Geometry: see drawing. Coordinates: mm, zero at the bounding-box minimum. Coordinates: 2 decimals unless noted, no trailing zeros. Loops run counter-clockwise (first coordinate to the right, second up) from the corner with the lowest first, then second, coordinate; pieces in that order, holes last.
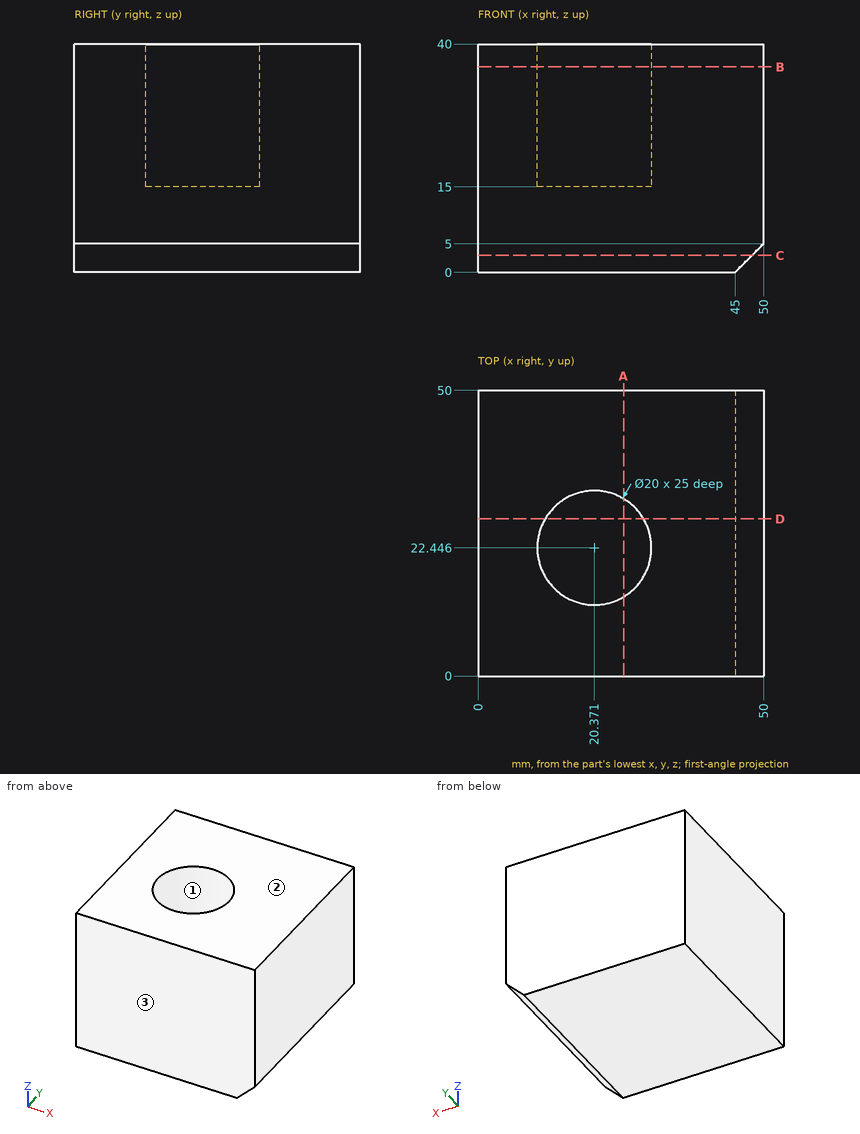
Item 1: Section query B-B (z = 36). Output: boundary loops of the cut face in (x, y) (1 decimal), then the cut area to 3 significant figures.
Result:
outline: (0, 0) - (50, 0) - (50, 50) - (0, 50) - close; hole circle Ø20 at (20.4, 22.4)
area: 2,190 mm2
Item 2: Section query D-D (y = 27.5). Output: boundary loops of the cut face in (x, z), then the cut area to 3 significant figures.
Result:
outline: (0, 0) - (45, 0) - (50, 5) - (50, 40) - (29, 40) - (29, 15) - (11.74, 15) - (11.74, 40) - (0, 40) - close
area: 1,560 mm2
Item 3: Mould query, pull axis Y, two halves, no side actions, for the marked faces 1, 2 and 3. Classes: +Y half, -Y half, draft (parallel to the pull), parting line (faces both ways), or undercut.
Result:
face 1: undercut
face 2: draft
face 3: -Y half
Item 4: Contact query for a flat-ended pin moving along its axis: P1, Ø8, axis at x = 25, z = 25.5, coming from the -Y side. Output: stop coordinate, or through.
Result:
P1: stops at y = 0
Item 5: Section query C-C (z = 3). Output: boundary loops of the cut face in (x, y), then the cut area to 3 significant figures.
Result:
outline: (0, 0) - (48, 0) - (48, 50) - (0, 50) - close
area: 2,400 mm2
Item 6: Line query: L1, parallel to X at y = 20, z = 28.5 (1 decimal); L2, parallel to Z at x = 13, y = 16.5; L3, parallel to Y at x = 28.5, z = 38.5. Output: solid intervals per line, ascending.
Result:
L1: x = 0 to 10.7, 30.1 to 50
L2: z = 0 to 15
L3: y = 0 to 16.62, 28.27 to 50
Item 7: Section query A-A (x = 25.5). Output: boundary loops of the cut face in (y, z).
Result:
outline: (0, 0) - (50, 0) - (50, 40) - (31.03, 40) - (31.03, 15) - (13.86, 15) - (13.86, 40) - (0, 40) - close
